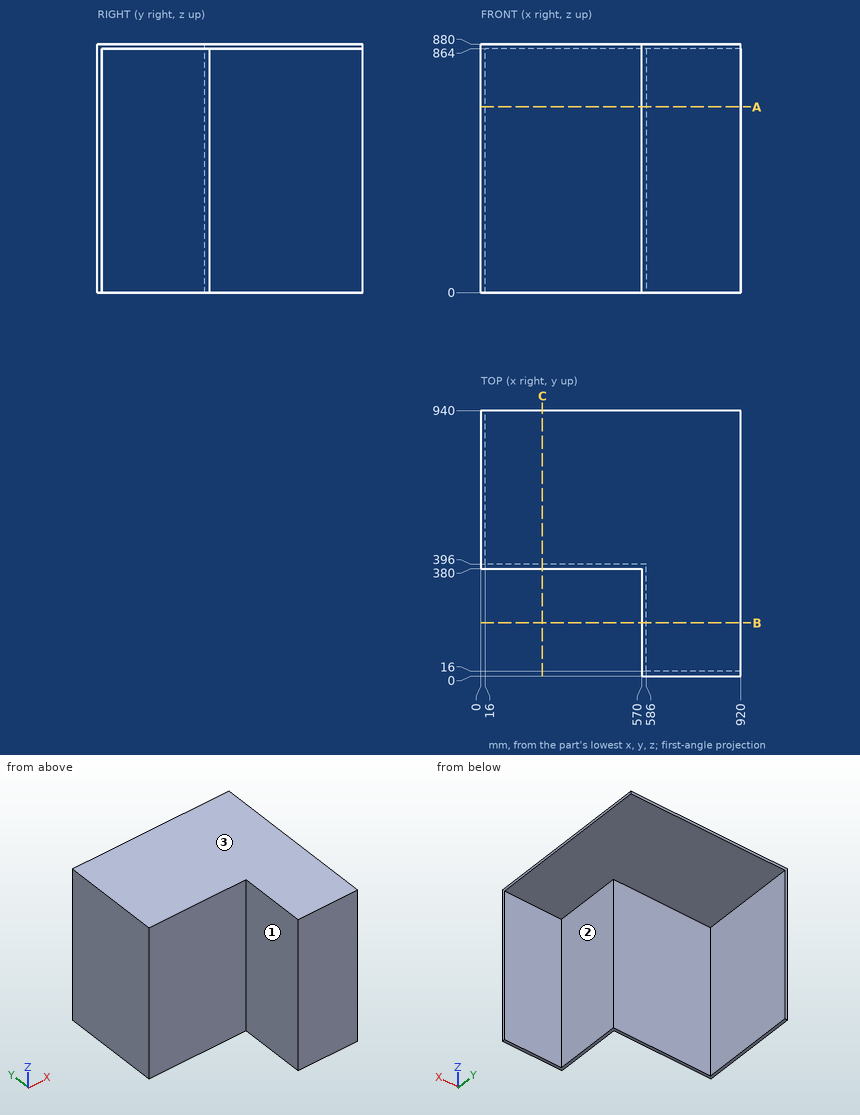
The drawing under review shows one solid part. Ordinate dimensions are in mm from its lowest x, y, z. A direction names the side the tool comes from. Round coordinates to 2 decimals unless told otherwise and drop trailing zeros. Write each loop counter-clockwise with the first axis right and the second up, starting at its lowest first coordinate (ties: lowest second). Pieces come first, ordered by that corner, then holes. Notation, with made-up numbers: M 34,77.25 L 57,77.25 A16 cw 57,104.25 Z; hole C 35.5,88 d7. An arc over 180 degrees is marked long. One line per item, written item: value. Start each with the question number.
(1) Wall thickness on line 1 (Z direction, x = 610.5, y = 188); line 2 (Y direction, x = 139.5, z = 514.5); line 3 (X direction, y = 726.5, z = 56): over which ranges is each line inside the solid? List them lowest first.
(2) We need section A-A (z = 657). Give the boundary of the cut face in (x, y).
(3) We need section B-B (y = 188). Give the boundary of the cut face in (x, z), and give its area (3 significant figures).
(4) Machinability: for the marked faces 1, 2 and 3, which of the approach directions +Z, -Z, +X, -X, +Y, -Y give a long, thin tool a straight path to every point of the face, cutting with its end or side? Answer none if there is none.
(5) Insertion check: pin 1 (2 mm diameter, centred on y = 461, z = 159.5, fed in from +X); pin 2 (6 mm diameter, centred on x = 765, z = 230.5, fed in from +Y); pin 3 (2 mm diameter, centred on x = 131, y = 536.5, fed in from -Z). Each pin has a flat end and moves straight along its axis. Give the tip position at first contact, or say it passes through.
(6) We need section C-C (x = 218). Give the boundary of the cut face in (y, z).
Result:
1. line 1: 864 to 880
1. line 2: 380 to 396
1. line 3: 0 to 16
2. outline: M 0,380 L 570,380 L 570,0 L 920,0 L 920,16 L 586,16 L 586,396 L 16,396 L 16,940 L 0,940 Z
3. outline: M 570,0 L 586,0 L 586,864 L 920,864 L 920,880 L 570,880 Z
3. area: 19,400 mm²
4. face 1: +Z, -Z, -X, -Y
4. face 2: -Z, +X, +Y
4. face 3: +Z, +X, -X, +Y, -Y
5. pin 1: x = 16
5. pin 2: y = 16
5. pin 3: z = 864
6. outline: M 380,0 L 396,0 L 396,864 L 940,864 L 940,880 L 380,880 Z
